The model under review builds one solid part; all positions refer to its coordinate system, in mm. Coordinates: 2 decimals unless noted, no trailing zeros. Answer as a JSON object with one key per item and string values.
```python
from build123d import *

# Parameters (mm, degrees)
BOSS_EXTRUDE1_DEPTH                               = 3
CSK_FOR_1_FLAT_HEAD_MACHINE_SCREW_100_D           = 2.0574
CSK_FOR_1_FLAT_HEAD_MACHINE_SCREW_100_CSINK_D     = 3.7084
CSK_FOR_1_FLAT_HEAD_MACHINE_SCREW_100_CSINK_ANGLE = 100


with BuildPart() as part:
    # Sketch1 → Boss-Extrude1 (new body)
    with BuildSketch(Plane.YZ):
        with BuildLine():
            Line((-70.802499273, 22.065445977), (-70.802499273, -19.520741015))
            ThreePointArc((-70.802499273, -19.520741015), (-70.170142814, -21.047384555), (-68.643499273, -21.679741015))
            Line((-68.643499273, -21.679741015), (68.643499273, -21.679741015))
            ThreePointArc((68.643499273, -21.679741015), (70.170142814, -21.047384555), (70.802499273, -19.520741015))
            Line((70.802499273, -19.520741015), (70.802499273, 22.065445977))
            ThreePointArc((70.802499273, 22.065445977), (70.170142814, 23.592089518), (68.643499273, 24.224445977))
            Line((68.643499273, 24.224445977), (-68.643499273, 24.224445977))
            ThreePointArc((-68.643499273, 24.224445977), (-70.170142814, 23.592089518), (-70.802499273, 22.065445977))
        make_face()
    extrude(amount=BOSS_EXTRUDE1_DEPTH)

    # CSK for #1 Flat Head Machine Screw (100)1 (through all)
    with Locations(Plane.YZ.offset(3)):
        with Locations((68.643499273, 22.065445977), (68.643499273, -19.520741015), (-68.643499273, -19.520741015), (-68.643499273, 22.065445977)):
            CounterSinkHole(CSK_FOR_1_FLAT_HEAD_MACHINE_SCREW_100_D / 2, CSK_FOR_1_FLAT_HEAD_MACHINE_SCREW_100_CSINK_D / 2, counter_sink_angle=CSK_FOR_1_FLAT_HEAD_MACHINE_SCREW_100_CSINK_ANGLE)


solid = part.part
```
(1) For pin 1 Ø2.5 at (y, z) = (68.64, 22.07) entering from -X; pin 2 Ø2.5 at (y, z) = (-68.64, 22.07) entering from +X, all flat-tipped, find the tip position at first contact; note any pin that passes through.
Results list:
{"pin 1": "x = 0", "pin 2": "x = 2.5"}
(2) Wall thickness on line 1 along Y through (x, z) = (0.4, 21.5): over which ranges is the line inside the solid? List them lowest first. Write a range as from..to.
Results list:
{"line 1": "-70.8..-69.5, -67.78..67.78, 69.5..70.8"}
(3) Draft analysis for pull direction Y (two halves, no side actions). For faces 1 (the face through (1, 70.802, 1)), 2 (the face through (1, 1, 24.224)), 3 (the face through (1, -70.802, 2)), state which applies: released by +Y, released by -Y, zero draft, split by the parting line, or undercut.
Results list:
{"face 1": "released by +Y", "face 2": "zero draft", "face 3": "released by -Y"}
